Model file for the job. Use its own axes, mm. Coordinates: 2 decimals unless noted, no trailing zeros. Loops run counter-clockwise (first coordinate to the right, second up) from the corner with the lowest first, then second, coordinate; pieces in that order, holes last.
from build123d import *

# Parameters (mm, degrees)
SKETCH1_R           = 49.5046
BOSS_EXTRUDE1_DEPTH = 3.175
SKETCH2_R           = 47.6885
BOSS_EXTRUDE2_DEPTH = 3.175
SKETCH3_R           = 6.35
SKETCH3_R_2         = 3.175
SKETCH3_R_3         = 11.1125
SKETCH3_R_4         = 2.54
CUT_EXTRUDE1_DEPTH  = 71.297463271
BOSS_EXTRUDE3_START = -3.175
SKETCH4_R           = 49.5046
SKETCH4_R_2         = 47.6885
BOSS_EXTRUDE3_DEPTH = 3.175
SKETCH5_R           = 11.1125
BOSS_EXTRUDE4_DEPTH = 6.35
SKETCH6_R           = 2.54
BOSS_EXTRUDE5_DEPTH = 6.35


with BuildPart() as part:
    # Sketch1 → Boss-Extrude1 (new body)
    with BuildSketch(Plane.XY):
        Circle(SKETCH1_R)
    extrude(amount=BOSS_EXTRUDE1_DEPTH)

    # Sketch2 → Boss-Extrude2 (add)
    with BuildSketch(Plane.XY.offset(3.175)):
        Circle(SKETCH2_R)
    extrude(amount=BOSS_EXTRUDE2_DEPTH)

    # Sketch3 → Cut-Extrude1 (cut, through all)
    with BuildSketch(Plane.XY.offset(6.35)):
        with Locations((-12.7, -31.235352443)):
            Circle(SKETCH3_R)
        with Locations((12.7, -31.235352443)):
            Circle(SKETCH3_R)
        with Locations((-34.925, 0)):
            Circle(SKETCH3_R_2)
        with Locations((34.925, 0)):
            Circle(SKETCH3_R_2)
        with Locations((0, 6.35)):
            Circle(SKETCH3_R_3)
        with Locations((-14.850390051, -11.029456704)):
            Circle(SKETCH3_R_2)
        with Locations((-23.622, 29.972)):
            Circle(SKETCH3_R_4)
        with Locations((23.622, 29.972)):
            Circle(SKETCH3_R_4)
        with Locations((23.622, -17.272)):
            Circle(SKETCH3_R_4)
        with Locations((-23.622, -17.272)):
            Circle(SKETCH3_R_4)
    extrude(amount=-CUT_EXTRUDE1_DEPTH, mode=Mode.SUBTRACT)

    # Sketch4 → Boss-Extrude3 (add)
    with BuildSketch(Plane.XY.offset(6.35).offset(BOSS_EXTRUDE3_START)):
        Circle(SKETCH4_R)
        Circle(SKETCH4_R_2, mode=Mode.SUBTRACT)
    extrude(amount=BOSS_EXTRUDE3_DEPTH)

    # Sketch5 → Boss-Extrude4 (add)
    with BuildSketch(Plane.XY.offset(6.35)):
        with Locations((0, 6.35)):
            Circle(SKETCH5_R)
    extrude(amount=-BOSS_EXTRUDE4_DEPTH)

    # Sketch6 → Boss-Extrude5 (add)
    with BuildSketch(Plane.XY.offset(6.35)):
        with Locations((-23.622, -17.272)):
            Circle(SKETCH6_R)
        with Locations((23.622, -17.272)):
            Circle(SKETCH6_R)
    extrude(amount=-BOSS_EXTRUDE5_DEPTH)


solid = part.part
Q1. Drill centre lines: line 1 (X direction, y = -31.5, z = 4.25); line 2 (X direction, y = -26, z = 2.5); line 3 (Y direction, x = -12.7, z = 5). Where is each one in solid material? Low to high.
Answers:
line 1: x = -38.19 to -19.04, -6.36 to 6.36, 19.04 to 38.19
line 2: x = -42.13 to -16.29, -9.11 to 9.11, 16.29 to 42.13
line 3: y = -47.85 to -37.59, -24.89 to -13.37, -8.69 to 47.85
Q2. Mould opens along X. For faces 1 (the cylindrical face through (-6.445, 49.083, 3.131)), 2 (the flat face through (-1, 1, 6.35)), 3 (the cylindrical face through (-18.022, -10.89, 3.219)) say: +X half, -X half, draft (parallel to the pull), parting line (faces both ways), or undercut.
Answers:
face 1: parting line
face 2: draft
face 3: undercut
Q3. Flat gauge pins, fed straight in: P1, Ø2, axis at y = 39, z = 1, coming from the -X side; P2, Ø1.5, axis at x = 9.5, z = 4, coming from the +Y side; P3, Ø2, axis at y = -36, z = 4, coming from the -X side. Where does each tip first touch, or does it go through?
Answers:
P1: stops at x = -31.73
P2: stops at y = 48.73
P3: stops at x = -35.01
Q4. Slice it at A-A (y = 0). List the corners of the cut face in (x, z).
Answers:
outline: (-49.5, 0) - (-38.1, 0) - (-38.1, 6.35) - (-49.5, 6.35) - close; (-31.75, 0) - (31.75, 0) - (31.75, 6.35) - (-31.75, 6.35) - close; (38.1, 0) - (49.5, 0) - (49.5, 6.35) - (38.1, 6.35) - close
Q5. Slice it at C-C (z = 1.75). List the corners of the cut face in (x, y) (3 decimals).
Answers:
outline: circle Ø99.009 at (0, 0); hole circle Ø6.35 at (-34.925, 0); hole circle Ø5.08 at (-23.622, 29.972); hole circle Ø12.7 at (-12.7, -31.235); hole circle Ø6.35 at (-14.85, -11.029); hole circle Ø12.7 at (12.7, -31.235); hole circle Ø5.08 at (23.622, 29.972); hole circle Ø6.35 at (34.925, 0)
Q6. Slice it at D-D (x = 12.7). List the corners of the cut face in (y, z), and give its area (3 significant figures).
Answers:
outline: (-47.85, 0) - (-37.59, 0) - (-37.59, 6.35) - (-47.85, 6.35) - close; (-24.89, 0) - (47.85, 0) - (47.85, 6.35) - (-24.89, 6.35) - close
area: 527 mm2
Q7. Slice it at B-B (x = -16). List the corners of the cut face in (y, z), and give its area (3 significant figures).
Answers:
outline: (-46.85, 0) - (-36.66, 0) - (-36.66, 6.35) - (-46.85, 6.35) - close; (-25.81, 0) - (-13.99, 0) - (-13.99, 6.35) - (-25.81, 6.35) - close; (-8.07, 0) - (46.85, 0) - (46.85, 6.35) - (-8.07, 6.35) - close
area: 488 mm2
